Geometry: final body of the model. Coordinates: model frame, mm. Face numbers are marked on the shaded views. A direction names the side the tool comes from. Coordinates: 2 decimals unless noted, no trailing zeros. Loops run counter-clockwise (first coordinate to the right, second up) from the corner with the lowest first, then second, coordinate; pieces in that order, holes last. Notation, with made-up numbers: M 7.25,3.25 L 48.25,3.25 A12 cw 48.25,8.25 Z; hole C 61.5,-10 d9. An arc over 180 degrees is marked long. Write item = value, one per line. Start each with the question number.
```python
from build123d import *

# Parameters (mm, degrees)
BOSS_EXTRUDE1_DEPTH = 88
CUT_EXTRUDE1_DEPTH  = 227.934618696
SKETCH3_R           = 15
CUT_EXTRUDE2_DEPTH  = 227.934618696
SKETCH4_R           = 44
BOSS_EXTRUDE3_DEPTH = 50
SCALE1_SCALE        = 0.3


with BuildPart() as part:
    # Sketch1 → Boss-Extrude1 (new body)
    with BuildSketch(Plane.XY):
        Polygon((27.330348609, 81.508634223), (27.330348609, 59.807321306), (27.330348609, -59.807321306), (27.330348609, -80.491365777), (57.330348609, -80.491365777), (132.330348609, -80.491365777), (132.330348609, -52.491365777), (57.330348609, -52.491365777), (57.330348609, 53.508634223), (132.330348609, 53.508634223), (132.330348609, 81.508634223), (57.330348609, 81.508634223), align=None)
    extrude(amount=BOSS_EXTRUDE1_DEPTH)

    # Sketch2 → Cut-Extrude1 (cut, through all)
    with BuildSketch(Plane(origin=(0, 81.508634223, 0), x_dir=(1, 0, 0), z_dir=(0, 1, 0))):
        with BuildLine():
            Line((132.330348609, 0), (57.330348609, 0))
            Line((57.330348609, 0), (110.543103545, -15.146046088))
            ThreePointArc((110.543103545, -15.146046088), (126.271763021, -25.922149576), (132.330348609, -44))
            Line((132.330348609, -44), (132.330348609, 0))
        make_face()
        with BuildLine():
            Line((132.330348609, -88), (132.330348609, -44))
            ThreePointArc((132.330348609, -44), (126.271763021, -62.077850424), (110.543103545, -72.853953912))
            Line((110.543103545, -72.853953912), (57.330348609, -88))
            Line((57.330348609, -88), (132.330348609, -88))
        make_face()
    extrude(amount=-CUT_EXTRUDE1_DEPTH, mode=Mode.SUBTRACT)

    # Sketch3 → Cut-Extrude2 (cut, through all)
    with BuildSketch(Plane(origin=(0, 81.508634223, 0), x_dir=(1, 0, 0), z_dir=(0, 1, 0))):
        with Locations(Location((102.330348609, -44, 0), (0, 0, 180))):
            Circle(SKETCH3_R)
    extrude(amount=-CUT_EXTRUDE2_DEPTH, mode=Mode.SUBTRACT)

    # Sketch4 → Boss-Extrude3 (add)
    with BuildSketch(Plane.ZY.offset(-27.330348609)):
        with Locations((44, 0.508634223)):
            Circle(SKETCH4_R)
        with BuildLine():
            Line((24.404082058, 4.508634223), (20.404082058, 4.508634223))
            Line((20.404082058, 4.508634223), (20.404082058, -3.491365777))
            Line((20.404082058, -3.491365777), (24.404082058, -3.491365777))
            ThreePointArc((24.404082058, -3.491365777), (64, 0.508634223), (24.404082058, 4.508634223))
        make_face(mode=Mode.SUBTRACT)
    extrude(amount=BOSS_EXTRUDE3_DEPTH)


with BuildPart() as part_1:
    # Scale1: scaled about (43.08652806, 0.508634223, 44.036146931)
    add(part.part.scale(SCALE1_SCALE).moved(Location((30.160569642, 0.356043956, 30.825302852))))


solid = part_1.part
```
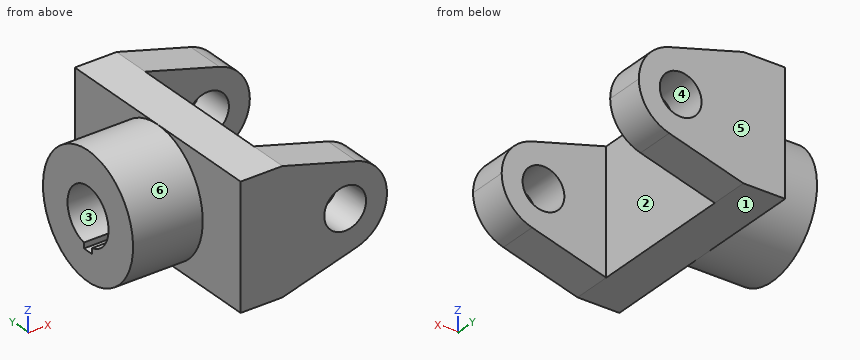
Item 1: Section query D-D (x = 59). Return the cut outline in (y, z).
Item 2: Pull-direction query (Z, two-part tool) for the marked faces 4, 5 and 6; classes: released by +Z, released by -Z, zero draft, split by the parting line, or undercut.
Item 3: Line query: line 1 (Y direction, x = 50.5, z = 36); line 2 (X direction, y = 3.5, z = 41.25); line 3 (Y direction, x = 25, z = 40.75). Output: solid intervals per line, ascending. Write a range as from..to.
Item 4: First-contact query: pin 1 (5 mm diameter, centred on x = 29.5, z = 50, fed in from -Y); pin 2 (7 mm diameter, centred on x = 60.86, z = 44.03, fed in from +Y); pin 3 (3 mm diameter, centred on y = 15.5, z = 40, fed in from -X); pin 4 (7 mm diameter, centred on y = 0.51, z = 44.03, fed in from +X). Flat tips, straight axial feed; report the tip coordinate or a pass-through.
Item 5: Reachability of the marked faces 1, 2 and 3 from +Z, -Z, +X, -X, +Y, -Y: full face, straight path, thin tool, end or side. Return the list, or none.
Item 6: Section query C-C (y = 8.5). Return the cut outline in (x, z), plus the area to 3 significant figures.
Item 7: Section query A-A (x = 50.5). Return the cut outline in (y, z), plus the area to 3 significant figures.
Item 8: Section query B-B (z = 43.25). Return the cut outline in (x, y).
Verdict:
q1.outline = M -23.79,34.14 L -15.39,34.14 L -15.39,39.93 L -23.79,39.93 Z; M -23.79,48.12 L -15.39,48.12 L -15.39,53.91 L -23.79,53.91 Z; M 16.41,34.14 L 24.81,34.14 L 24.81,39.93 L 16.41,39.93 Z; M 16.41,48.12 L 24.81,48.12 L 24.81,53.91 L 16.41,53.91 Z
q2.face_4 = undercut
q2.face_5 = zero draft
q2.face_6 = split by the parting line
q3.line_1 = -23.79..-15.39, 16.41..24.81
q3.line_2 = 38.36..47.36
q3.line_3 = -12.28..-4.52, 5.54..13.3
q4.pin_1 = -12.23
q4.pin_2 = through
q4.pin_3 = 38.36
q4.pin_4 = 47.36
q5.face_1 = -Z, +X, -X, +Y, -Y
q5.face_2 = +Z, -Z, +X
q5.face_3 = -X
q6.outline = M 23.36,33.52 L 38.36,33.52 L 38.36,30.83 L 47.36,30.83 L 47.36,57.23 L 38.36,57.23 L 38.36,54.53 L 23.36,54.53 Z
q6.area = 553 mm2
q7.outline = M -23.79,31.72 L -15.39,31.72 L -15.39,56.33 L -23.79,56.33 Z; M 16.41,31.72 L 24.81,31.72 L 24.81,56.33 L 16.41,56.33 Z
q7.area = 413 mm2
q8.outline = M 23.36,-12.67 L 38.36,-12.67 L 38.36,-23.79 L 56.43,-23.79 L 56.43,-15.39 L 47.36,-15.39 L 47.36,16.41 L 56.43,16.41 L 56.43,24.81 L 38.36,24.81 L 38.36,13.69 L 23.36,13.69 L 23.36,6.46 L 38.36,6.46 L 38.36,-5.44 L 23.36,-5.44 Z; M 65.29,-23.79 L 69.83,-23.79 L 69.83,-15.39 L 65.29,-15.39 Z; M 65.29,16.41 L 69.83,16.41 L 69.83,24.81 L 65.29,24.81 Z
